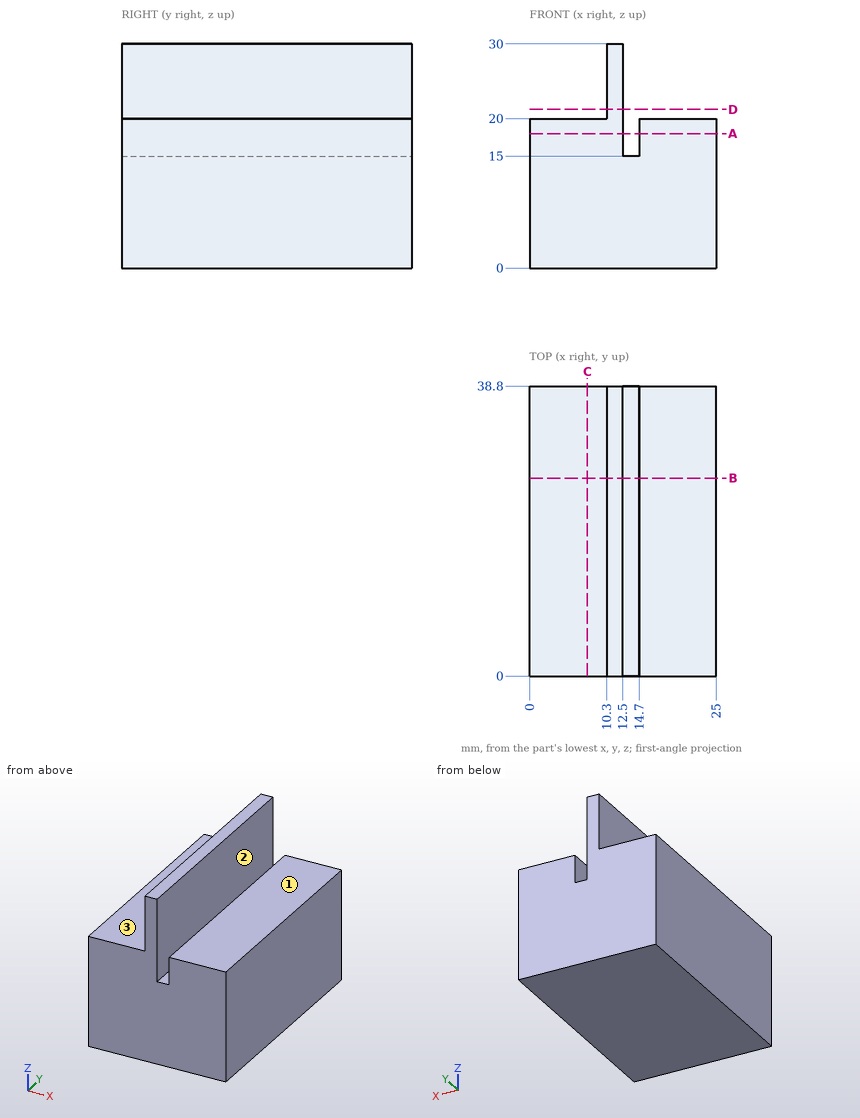
Could you check a few things on this drawing? It's one solid part, dimensions in mm from its lowest x, y, z. A direction names the side the tool comes from. Round coordinates to 2 decimals unless told otherwise and drop trailing zeros. Loops run counter-clockwise (first coordinate to the right, second up) from the corner with the lowest first, then second, coordinate; pieces in that order, holes last. Notation, with made-up numbers: M 68.25,19 L 127.25,19 A3 cw 127.25,23 Z; hole C -9.5,87.25 d2. An arc over 180 degrees is marked long. Write each question's results on one line, items separated by ' | '. Start each with the question number.
(1) I want a section at D-D (z = 21.25). Please give me the cut outline in (x, y), then the cut area to 3 significant figures.
(2) If I drill on probe 1 along X at (y, z) = (12, 18.5); probe 2 along Z at (x, y) = (3.25, 31); probe 3 along Z at (x, y) = (13.75, 13), over which ranges is the centre line in solid material (lowest first)? Write a range as from..to.
(3) I want a section at B-B (y = 26.5). Please give me the cut outline in (x, z).
(4) On a 3-axis mill with a long thin cutter (end or side, diameter ignored), from which of +Z, -Z, +X, -X, +Y, -Y can I reach the whole of each face in a straight line? I mean the marked faces 1, 2 and 3. Say none if no direction works.
(5) Will these pins go through, and if not, where does the flat tip stop? P1, Ø11.5, axis at x = 21, y = 12, coming from the +Z side; P2, Ø1.1, axis at x = 13.5, y = 26.5, coming from the +Z side; P3, Ø11, axis at y = 11.5, z = 26.5, coming from the -X side.
(6) I want a section at C-C (x = 7.75). Please give me the cut outline in (y, z).
(7) I want a section at A-A (z = 18). Please give me the cut outline in (x, y), then the cut area to 3 significant figures.
Solved:
1) outline: M 10.3,0 L 12.5,0 L 12.5,38.8 L 10.3,38.8 Z | area: 85.4 mm²
2) probe 1: x = 0..12.5, 14.7..25 | probe 2: z = 0..20 | probe 3: z = 0..15
3) outline: M 0,0 L 25,0 L 25,20 L 14.7,20 L 14.7,15 L 12.5,15 L 12.5,30 L 10.3,30 L 10.3,20 L 0,20 Z
4) face 1: +Z, +X, +Y, -Y | face 2: +Z, +Y, -Y | face 3: +Z, -X, +Y, -Y
5) P1: stops at z = 20 | P2: stops at z = 15 | P3: stops at x = 10.3
6) outline: M 0,0 L 38.8,0 L 38.8,20 L 0,20 Z
7) outline: M 0,0 L 12.5,0 L 12.5,38.8 L 0,38.8 Z; M 14.7,0 L 25,0 L 25,38.8 L 14.7,38.8 Z | area: 885 mm²
